Check sheet for the modelled part. Datum: model origin and axes. Units: mm. Face numbers are marked on the shaded views. Round coordinates to 2 decimals unless told otherwise and drop trailing zeros. Write each loop counter-clockwise with the first axis right and the second up, starting at its lowest first coordinate (ties: lowest second). Pieces come first, ordered by that corner, then holes.
Item 1: Cross-section at A-A on y = 1.5. Enter the section's corners in (x, z).
Item 2: Material ranges on line 1 (X direction, y = -0.25, z = 0); line 2 (Z direction, x = 0, y = 8.5); line 3 (Z direction, x = 6, y = -3), recorded low to high.
Item 3: Release check for a two-part mould opening along X. For the marked faces 1, 2, 3 and 4 record: +X half, -X half, draft (parallel to the pull), parting line (faces both ways), or undercut.
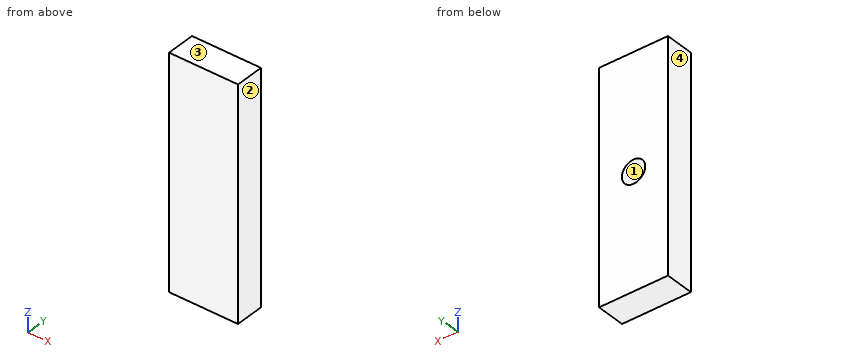
from build123d import *

# Parameters (mm, degrees)
SKETCH1_W                 = 76.2
SKETCH1_H                 = 31.75
BOSS_EXTRUDE1_DEPTH       = 127
F_1_CLEARANCE_HOLE1_D     = 25.79624
F_1_CLEARANCE_HOLE1_DEPTH = 24.003
F_1_CLEARANCE_HOLE1_TIP   = 7.749972367


with BuildPart() as part:
    # Sketch1 → Boss-Extrude1 (new body, symmetric)
    with BuildSketch(Plane.XY):
        Rectangle(SKETCH1_W, SKETCH1_H)
    extrude(amount=BOSS_EXTRUDE1_DEPTH, both=True)

    # 1 Clearance Hole1
    with Locations(Plane(origin=(0, 15.875, 0), x_dir=(-1, 0, 0), z_dir=(0, 1, 0))):
        with Locations((0, 0)):
            Hole(F_1_CLEARANCE_HOLE1_D / 2, depth=F_1_CLEARANCE_HOLE1_DEPTH)
            with Locations((0, 0, -(F_1_CLEARANCE_HOLE1_DEPTH + F_1_CLEARANCE_HOLE1_TIP / 2))):  # 118° drill point
                Cone(0, F_1_CLEARANCE_HOLE1_D / 2, F_1_CLEARANCE_HOLE1_TIP, mode=Mode.SUBTRACT)


solid = part.part
Response values:
1. outline: (-38.1, -127) - (38.1, -127) - (38.1, 127) - (-38.1, 127) - close; hole circle Ø25.8 at (0, 0)
2. line 1: x = -38.1 to -12.9, 12.9 to 38.1
2. line 2: z = -127 to -12.9, 12.9 to 127
2. line 3: z = -127 to -11.42, 11.42 to 127
3. face 1: undercut
3. face 2: +X half
3. face 3: draft
3. face 4: -X half
